Geometry check sheet. Reference: the model listing, model coordinates, mm. Face numbers are marked on the shaded views. A direction names the side the tool comes from. Coordinates: 2 decimals unless noted, no trailing zeros. Write each loop counter-clockwise with the first axis right and the second up, starting at its lowest first coordinate (ties: lowest second). Pieces come first, ordered by that corner, then holes. Notation, with made-up numbers: (23, 43) -> (59, 43) arc R6 cw to (59, 52) -> close; hole circle Ø10 at (-5, -4.75). An arc over 180 degrees is marked (long way). Use a Markdown table: item, result.
```python
from build123d import *

# Parameters (mm, degrees)
BOSS_EXTRUDE1_DEPTH = 10
SKETCH2_R           = 7
CUT_EXTRUDE1_DEPTH  = 5


with BuildPart() as part:
    # Sketch1 → Boss-Extrude1 (new body)
    with BuildSketch(Plane.XY):
        with BuildLine():
            Line((0, 0), (-15.642172524, 15.642172524))
            Line((-15.642172524, 15.642172524), (-4.089456869, 50.095846645))
            Line((-4.089456869, 50.095846645), (1.922169026, 48.080078912))
            Line((1.922169026, 48.080078912), (0, 19.833865815))
            Line((0, 19.833865815), (6.134185304, 13.699680511))
            Line((6.134185304, 13.699680511), (12.268370607, 19.833865815))
            Line((12.268370607, 19.833865815), (10.346201581, 48.080078912))
            Line((10.346201581, 48.080078912), (16.357827476, 50.095846645))
            Line((16.357827476, 50.095846645), (27.910543131, 15.642172524))
            Line((27.910543131, 15.642172524), (12.268370607, 0))
            Line((12.268370607, 0), (22.134185304, -65.230001967))
            ThreePointArc((22.134185304, -65.230001967), (6.134185304, -94.406570423), (-9.865814696, -65.230001967))
            Line((-9.865814696, -65.230001967), (0, 0))
        make_face()
    extrude(amount=BOSS_EXTRUDE1_DEPTH)

    # Sketch2 → Cut-Extrude1 (cut)
    with BuildSketch(Plane.XY.offset(10)):
        with Locations((6.134185304, -75.431204137)):
            Circle(SKETCH2_R)
    extrude(amount=-CUT_EXTRUDE1_DEPTH, mode=Mode.SUBTRACT)


solid = part.part
```
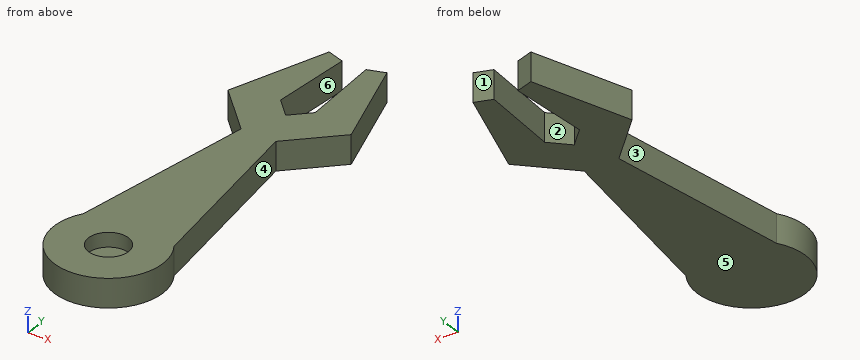
Item 1: Section check C-C on x = 8. Record the boundary of the cut face in (y, z).
Answer block:
| item | result |
|---|---|
| outline | (-94.31, 0) -> (15.57, 0) -> (15.57, 10) -> (-68.68, 10) -> (-68.68, 5) -> (-82.18, 5) -> (-82.18, 10) -> (-94.31, 10) -> close |
Item 2: Mould release check, pull along X, two halves, no side actions. Record for the marked faces 4, 5 and 6: +X half, -X half, draft (parallel to the pull), parting line (faces both ways), or undercut.
Answer block:
| item | result |
|---|---|
| face 4 | +X half |
| face 5 | draft |
| face 6 | undercut |
Item 3: Section check B-B on y = 31. Record the boundary of the cut face in (x, z), then the cut area to 3 significant figures.
Answer block:
| item | result |
|---|---|
| outline | (-10.49, 0) -> (0.76, 0) -> (0.76, 10) -> (-10.49, 10) -> close; (11.51, 0) -> (22.76, 0) -> (22.76, 10) -> (11.51, 10) -> close |
| area | 225 mm^2 |
Item 4: Depth check by flat-ended pin: P1, Ø3, axis at x = 7, z = 2, coming from the +Y side; P2, Ø6, axis at x = 2, z = 6.5, coming from the +Y side; P3, Ø1.5, axis at y = -35, z = 6.5, coming from the -X side. Enter the tip coordinate at first touch or a pass-through.
Answer block:
| item | result |
|---|---|
| P1 | stops at y = 16.07 |
| P2 | stops at y = 49.06 |
| P3 | stops at x = -5.41 |
Item 5: Tool access check on the marked faces 1, 2 and 3. Record the directions out of +Z, -Z, +X, -X, +Y, -Y that give a thin tool (end or side, any length) a straight path to the whole face; none if there is none.
Answer block:
| item | result |
|---|---|
| face 1 | +Z, -Z, +Y |
| face 2 | +Z, -Z |
| face 3 | +Z, -Z, -X |
Item 6: Section check D-D on y = -55. Record the boundary of the cut face in (x, z).
Answer block:
| item | result |
|---|---|
| outline | (-8.32, 0) -> (20.59, 0) -> (20.59, 10) -> (-8.32, 10) -> close |
Item 7: Thickness scan on L1, parallel to X at y = 21.5, z = 8.5; L2, parallel to Y at x = 2.5, z = 6; L3, parallel to X at y = 32.5, z = 1.75. Record the ranges inside material, lowest first. Write a range as [from, to].
Answer block:
| item | result |
|---|---|
| L1 | x = [-13.68, 0.11], [12.15, 25.95] |
| L2 | y = [-94.06, -81.41], [-69.45, 17.33] |
| L3 | x = [-9.99, 0.86], [11.41, 22.26] |
Item 8: Section check A-A on z = 3.5. Record the boundary of the cut face in (x, y).
Answer block:
| item | result |
|---|---|
| outline | (-15.64, 15.64) -> (0, 0) -> (-9.87, -65.23) arc R18.98 ccw (long way) to (22.13, -65.23) -> (12.27, 0) -> (27.91, 15.64) -> (16.36, 50.1) -> (10.35, 48.08) -> (12.27, 19.83) -> (6.13, 13.7) -> (0, 19.83) -> (1.92, 48.08) -> (-4.09, 50.1) -> close |
